Geometry: final body of the model. Coordinates: model frame, mm. A direction names the side the tool comes from. Give positions to 0.01 mm unless a question says otherwise; leave off trailing zeros. Write each loop counter-clockwise with the first axis right and the second up, starting at its lowest first coordinate (ties: lowest second). Pieces come first, ordered by that corner, then holes. Notation, with made-up numbers: (-22, 62) - (-6, 62) arc R30 cw to (-6, 99) - close; hole circle Ø7 at (71, -3). An arc over 180 degrees is marked (long way). Use CSV: the item, a comma, the result in double quotes. Start each with the question number.
(1) Reachability of faces 4 (the flat face through (-14.15, 2, 16)), 5 (the flat face through (0, 5, 10.6)) from +Z, -Z, +X, -X, +Y, -Y: full face, straight path, thin tool, end or side. Return the list, or none.
(2) Draft query along Z for faces 1 (the flat face through (0, 5, 7)), 2 (the flat face through (16, 0, -3)), 3 (the flat face through (5.1, 5, 9)). Return one class per face: released by +Z, released by -Z, zero draft, split by the parting line, or undercut.
(3) Section D-D on z = -15.5. Output: boundary loops of the cut face in (x, y).
(4) Section C-C on x = -8. Output: boundary loops of the cut face in (y, z).
(5) Section B-B on y = 2.6. Output: boundary loops of the cut face in (x, z).
(6) Line query: probe 1 along Z at (x, y) = (0, 5.15); probe 2 along X at (y, z) = (4.4, 0); probe 3 along X at (y, z) = (3.65, 0). Output: solid intervals per line, ascending. Write a range as [from, to].
(7) First-contact query: pin 1 Ø2 at (x, y) = (-1.5, 5) entering from -Z; pin 2 Ø1.6 at (x, y) = (8.5, 5.5) entering from -Z; pin 3 Ø1 at (y, z) = (5, -9.5) entering from +X. Flat tips, straight axial feed; report the tip coordinate or a pass-through.
(8) Section A-A on x = 0. Output: boundary loops of the cut face in (y, z).
from build123d import *

# Parameters (mm, degrees)
BOSS_EXTRUDE1_DEPTH = 6
SKETCH2_W           = 28.3
SKETCH2_H           = 64.3
CUT_EXTRUDE1_DEPTH  = 4
SKETCH3_R           = 1.45
SKETCH3_W           = 10.2
SKETCH3_H           = 3.6
CUT_EXTRUDE2_DEPTH  = 7
CIRPATTERN1_COUNT   = 4
CUT_EXTRUDE3_REACH  = 72.24
SKETCH4_W           = 25
SKETCH4_H           = 4


with BuildPart() as part:
    # Sketch1 → Boss-Extrude1 (new body)
    with BuildSketch(Plane(origin=(0, 0, 0), x_dir=(1, 0, 0), z_dir=(0, 1, 0))):
        with BuildLine():
            Line((-17.5, -32.939945355), (17.5, -32.939945355))
            ThreePointArc((17.5, -32.939945355), (0, 37.3), (-17.5, -32.939945355))
        make_face()
    extrude(amount=BOSS_EXTRUDE1_DEPTH)

    # Sketch2 → Cut-Extrude1 (cut)
    with BuildSketch(Plane.XZ):
        with Locations((0, -0.710054645)):
            Rectangle(SKETCH2_W, SKETCH2_H)
    extrude(amount=-CUT_EXTRUDE1_DEPTH, mode=Mode.SUBTRACT)

    # Sketch3 → Cut-Extrude2 (cut, through all)
    with BuildSketch(Plane(origin=(0, 6, 0), x_dir=(1, 0, 0), z_dir=(0, 1, 0))):
        with Locations((0, 15.5)):
            Circle(SKETCH3_R)
        with Locations((0, 8.8)):
            Rectangle(SKETCH3_W, SKETCH3_H)
    cut_extrude2 = extrude(amount=-CUT_EXTRUDE2_DEPTH, mode=Mode.SUBTRACT)

    # CirPattern1: Cut-Extrude2 ×4 about axis
    cirpattern1_axis = Axis((0, 0, 0), (0, 1, 0))
    for i in range(1, CIRPATTERN1_COUNT):
        add(cut_extrude2.rotate(cirpattern1_axis, i * 360 / CIRPATTERN1_COUNT), mode=Mode.SUBTRACT)

    # Sketch4 → Cut-Extrude3 (cut, up to next)
    with BuildSketch(Plane.XY.offset(32.939945355), mode=Mode.PRIVATE) as cut_extrude3_sk1:
        with Locations((0, 2)):
            Rectangle(SKETCH4_W, SKETCH4_H)
    cut_extrude3_tool1 = extrude(cut_extrude3_sk1.sketch, amount=-CUT_EXTRUDE3_REACH, mode=Mode.PRIVATE) & part.part
    add(cut_extrude3_tool1.solids().sort_by_distance((0, 2, 32.939945))[0], mode=Mode.SUBTRACT)


solid = part.part
Check values:
1,face 4,"-Y"
1,face 5,"+Y, -Y"
2,face 1,"undercut"
2,face 2,"zero draft"
2,face 3,"undercut"
3,outline,"(-33.93, 0) - (-14.15, 0) - (-14.15, 4) - (-1.45, 4) - (-1.45, 6) - (-33.93, 6) - close; (1.45, 4) - (14.15, 4) - (14.15, 0) - (33.93, 0) - (33.93, 6) - (1.45, 6) - close"
4,outline,"(0, -36.43) - (6, -36.43) - (6, -5.1) - (4, -5.1) - (4, -32.86) - (0, -32.86) - close; (4, 5.1) - (6, 5.1) - (6, 32.94) - (4, 32.94) - close"
5,outline,"(-17.5, 32.94) arc R37.3 ccw (long way) to (17.5, 32.94) - (12.5, 32.94) - (12.5, 31.44) - (14.15, 31.44) - (14.15, 0.53) arc R1.45 cw (long way) to (14.15, -0.53) - (14.15, -32.86) - (-14.15, -32.86) - (-14.15, -0.53) arc R1.45 cw (long way) to (-14.15, 0.53) - (-14.15, 31.44) - (-12.5, 31.44) - (-12.5, 32.94) - close"
6,probe 1,"z = [-37.3, -16.95], [-14.05, -10.6], [-7, 7], [10.6, 14.05], [16.95, 32.94]"
6,probe 2,"x = [-37.3, -16.95], [-14.05, -10.6], [-7, 7], [10.6, 14.05], [16.95, 37.3]"
6,probe 3,"x = [-37.3, -16.95], [16.95, 37.3]"
7,pin 1,"stops at z = -37.3"
7,pin 2,"stops at z = -36.5"
7,pin 3,"stops at x = 36.2"
8,outline,"(0, -37.3) - (6, -37.3) - (6, -16.95) - (4, -16.95) - (4, -32.86) - (0, -32.86) - close; (4, -14.05) - (6, -14.05) - (6, -10.6) - (4, -10.6) - close; (4, -7) - (6, -7) - (6, 7) - (4, 7) - close; (4, 10.6) - (6, 10.6) - (6, 14.05) - (4, 14.05) - close; (4, 16.95) - (6, 16.95) - (6, 32.94) - (4, 32.94) - close"
